Read the model definition and answer for the solid it produces. Units are mm, in the model's axes. A direction names the side the tool comes from. Round coordinates to 2 decimals unless told otherwise and drop trailing zeros. Write each loop counter-clockwise with the first axis right and the second up, starting at its lowest first coordinate (ties: lowest second). Pieces come first, ordered by that corner, then holes.
from build123d import *

# Parameters (mm, degrees)
F1_DEPTH = 25


with BuildPart() as f1:
    # F0 (on Front) → F1 (new body)
    with BuildSketch(Plane.XZ):
        with BuildLine():
            Line((0, 0), (0, 1.3))
            Line((0, 1.3), (-35.3, 1.3))
            Line((-35.3, 1.3), (-35.3, 5.6))
            Line((-35.3, 5.6), (-47.8, 5.6))
            Line((-47.8, 5.6), (-47.8, 1.3))
            Line((-47.8, 1.3), (-54, 1.3))
            ThreePointArc((-54, 1.3), (-56.616295, 2.383705), (-57.7, 5))
            Line((-57.7, 5), (-57.7, 16.5))
            Line((-57.7, 16.5), (-54.23428, 16.5))
            ThreePointArc((-54.23428, 16.5), (-52.133155, 14.514057), (-49.307358, 15.125262))
            ThreePointArc((-49.307358, 15.125262), (-49.22416, 16.076224), (-50.175122, 16.159422))
            ThreePointArc((-50.175122, 16.159422), (-53.05, 17.5), (-50.175122, 18.840578))
            ThreePointArc((-50.175122, 18.840578), (-49.22416, 18.923776), (-49.307358, 19.874738))
            ThreePointArc((-49.307358, 19.874738), (-52.133155, 20.485943), (-54.23428, 18.5))
            Line((-54.23428, 18.5), (-57.7, 18.5))
            Line((-57.7, 18.5), (-57.7, 24.3))
            Line((-57.7, 24.3), (-53.8, 24.3))
            Line((-53.8, 24.3), (-53.8, 23.1))
            Line((-53.8, 23.1), (-50.8, 23.1))
            Line((-50.8, 23.1), (-50.8, 24.3))
            Line((-50.8, 24.3), (-52.3, 24.3))
            Line((-52.3, 24.3), (-52.3, 26.3))
            Line((-52.3, 26.3), (-50.8, 26.3))
            Line((-50.8, 26.3), (-50.8, 27.5))
            Line((-50.8, 27.5), (-53.8, 27.5))
            Line((-53.8, 27.5), (-53.8, 26.3))
            Line((-53.8, 26.3), (-57.7, 26.3))
            Line((-57.7, 26.3), (-57.7, 30))
            Line((-57.7, 30), (-52.3, 30))
            ThreePointArc((-52.3, 30), (-51.8, 30.5), (-52.3, 31))
            Line((-52.3, 31), (-55, 31))
            Line((-55, 31), (-55, 33.7))
            Line((-55, 33.7), (-48.447221, 33.7))
            ThreePointArc((-48.447221, 33.7), (-47.801861, 34.250918), (-48.352779, 34.896278))
            Line((-48.352779, 34.896278), (-52.2, 35.2))
            Line((-52.2, 35.2), (-54, 35.2))
            ThreePointArc((-54, 35.2), (-57.535534, 33.735534), (-59, 30.2))
            Line((-59, 30.2), (-59, 5))
            ThreePointArc((-59, 5), (-57.535534, 1.464466), (-54, 0))
            Line((-54, 0), (-44.85, 0))
            ThreePointArc((-44.85, 0), (-44.2, 0.65), (-44.85, 1.3))
            Line((-44.85, 1.3), (-46.6, 1.3))
            Line((-46.6, 1.3), (-46.6, 4.4))
            Line((-46.6, 4.4), (-36.5, 4.4))
            Line((-36.5, 4.4), (-36.5, 1.3))
            Line((-36.5, 1.3), (-38.25, 1.3))
            ThreePointArc((-38.25, 1.3), (-38.9, 0.65), (-38.25, 0))
            Line((-38.25, 0), (0, 0))
        make_face()
    extrude(amount=F1_DEPTH)

    # F2: F1 across plane


with BuildPart() as f1_1:
    add(f1.part)
    add(f1.part.mirror(Plane.YZ))


solid = f1_1.part
Q1. Straight lines are drawn through the part: probe 1 along X at (y, z) = (-9.5, 23.5); probe 2 along X at (y, z) = (-9, 17.5); probe 3 along X at (y, z) = (-4.5, 5). For each, find the intervals that lie inside material, in ascending order.
Verdict:
probe 1: x = -59 to -57.7, -53.8 to -50.8, 50.8 to 53.8, 57.7 to 59
probe 2: x = -59 to -53.05, 53.05 to 59
probe 3: x = -59 to -57.7, -47.8 to -35.3, 35.3 to 47.8, 57.7 to 59
Q2. Section A-A (z = 2.5) is taken. Determine the outline of the cut face in (x, y), then the cut area to 3 significant figures.
Verdict:
outline: (-58.33, -25) - (-56.73, -25) - (-56.73, 0) - (-58.33, 0) - close; (-47.8, -25) - (-46.6, -25) - (-46.6, 0) - (-47.8, 0) - close; (-36.5, -25) - (-35.3, -25) - (-35.3, 0) - (-36.5, 0) - close; (35.3, -25) - (36.5, -25) - (36.5, 0) - (35.3, 0) - close; (46.6, -25) - (47.8, -25) - (47.8, 0) - (46.6, 0) - close; (56.73, -25) - (58.33, -25) - (58.33, 0) - (56.73, 0) - close
area: 200 mm2
Q3. Flat-ended cylindrical pins translate along their axes: pin 1 Ø6 at (y, z) = (-18.5, 31) entering from -X; pin 2 Ø1.5 at (x, y) = (30.5, -6) entering from +Z; pin 3 Ø1.4 at (x, y) = (-46, -9) entering from +Z; pin 4 Ø3 at (x, y) = (-56.5, -7.5) entering from +Z. Find the tip coordinate at first contact, or state that the pin passes through.
Verdict:
pin 1: stops at x = -59
pin 2: stops at z = 1.3
pin 3: stops at z = 5.6
pin 4: stops at z = 35.1
Q4. Determine the mould class of faces 3 (the flat face through (59, -12, 18)), 4 (the flat face through (0, -25, 1)), 5 (the cylindrical face through (-58, -12, 2)), 6 (the flat face through (46.6, -12, 3)) for opening direction X: pulls with the +X half, pulls with the -X half, needs draft (parallel to the pull), parting line crosses it, or undercut.
Verdict:
face 3: pulls with the +X half
face 4: needs draft
face 5: pulls with the -X half
face 6: undercut
Q5. Which of the six approach directions +Z, -Z, +X, -X, +Y, -Y give full straight-line access (tool end or side, diameter ignored) to faces 1 (the flat face through (-41, -12, 5.6)), 2 (the flat face through (-56, -12, 26.3))?
Verdict:
face 1: +Z, +Y, -Y
face 2: +Y, -Y
Q6. Section B-B (x = -18) is taken. Determine the outline of the cut face in (y, z), then the cut area to 3 significant figures.
Verdict:
outline: (-25, 0) - (0, 0) - (0, 1.3) - (-25, 1.3) - close
area: 32.5 mm2
